Check sheet for the modelled part. Datum: model origin and axes. Units: mm. A direction names the side the tool comes from. Round coordinates to 2 decimals unless told otherwise and drop trailing zeros. Write each loop counter-clockwise with the first axis right and the second up, starting at its lowest first coordinate (ties: lowest second). Pieces come first, ordered by that corner, then holes.
Item 1: Tool access check on faces 5 (the flat face through (-44, 66, -115)), 6 (the flat face through (2, 173, 115)), 7 (the flat face through (-195.247, -51.359, 90.437)), 8 (the flat face through (195.247, -50.911, 90.437)), 9 (the flat face through (2.381, -89.352, 84.531)). Record the directions out of +Z, -Z, +X, -X, +Y, -Y that give a thin tool (end or side, any length) a straight path to the whole face; none if there is none.
Item 2: Go/stop test with flat-tipped pins: pin 1 Ø12 at (y, z) = (275, -32.5) entering from -X; pin 2 Ø6 at (y, z) = (141.5, 30.5) entering from +X; pin 3 Ø11.5 at (x, y) = (-20.5, -47) entering from +Z. Record where each tip stops, or that it passes through.
Item 3: Material ranges on line 1 (Y direction, x = 0, z = -46); line 2 (X direction, y = -46, z = -49); line 3 (Z direction, x = -53.5, y = -56), recorded low to high.
Item 4: Cross-section at D-D on z = 44.5. Enter the section's corners in (x, y), plus the area to 3 significant figures.
Item 5: Cross-section at B-B on z = -22.5. Enter the section's corners in (x, y), plus the area to 3 significant figures.
Item 6: Cross-section at A-A on z = -49. Enter the section's corners in (x, y), plus the area to 3 significant figures.
Item 7: Cross-section at C-C on z = 88. Enter the section's corners in (x, y).
Item 8: Release check for a two-part mould opening along X. For faces 1 (the flat face through (2, -110.03, -25)), 2 (the cylindrical face through (-205.024, -95.772, -25.479)), 3 (the flat face through (225.06, 39, 53)), 4 (the cylindrical face through (10.84, 61.22, -65.7)) record: +X half, -X half, draft (parallel to the pull), parting line (faces both ways), or undercut.
from build123d import *
from OCP.BRepFilletAPI import BRepFilletAPI_MakeChamfer

# Parameters (mm, degrees)
BOSS_EXTRUDE1_DEPTH = 115
CHAMFER3_SIZE       = 60
CHAMFER3_SIZE2      = 42.012452293
FILLET1_R           = 10
SKETCH2_R           = 88.57
BOSS_EXTRUDE2_DEPTH = 225.06
SKETCH3_R           = 50
CUT_EXTRUDE1_DEPTH  = 100


with BuildPart() as part:
    # Sketch1 → Boss-Extrude1 (new, symmetric)
    with BuildSketch(Plane.XY):
        with BuildLine():
            ThreePointArc((-220.06, 110.03), (0, 330.09), (220.06, 110.03))
            Line((220.06, 110.03), (-220.06, 110.03))
        make_face()
        with BuildLine():
            ThreePointArc((-170.06, -110.03), (-205.415339059, -95.385339059), (-220.06, -60.03))
            Line((-220.06, -60.03), (-220.06, 110.03))
            Line((-220.06, 110.03), (220.06, 110.03))
            Line((220.06, 110.03), (220.06, -60.03))
            ThreePointArc((220.06, -60.03), (205.415339059, -95.385339059), (170.06, -110.03))
            Line((170.06, -110.03), (-170.06, -110.03))
        make_face()
    extrude(amount=BOSS_EXTRUDE1_DEPTH, both=True)

    # Chamfer3: one chamfer whose edges measure the first distance from different faces: ONE call of the kernel's chamfer builder (chamfer() names one face for all edges)
    chamfer3_edges_1 = [part.edges().sort_by_distance(p)[0] for p in [
        (-220.06, 25, 115),
    ]]
    chamfer3_side_1 = [part.faces().sort_by_distance(p)[0] for p in [
        (-220.06, 25, 0),
    ]]
    chamfer3_edges_2 = [part.edges().sort_by_distance(p)[0] for p in [
        (-205.415339059, -95.385339059, 115),
    ]]
    chamfer3_side_2 = [part.faces().sort_by_distance(p)[0] for p in [
        (-205.415339059, -95.385339059, 0),
    ]]
    chamfer3_edges_3 = [part.edges().sort_by_distance(p)[0] for p in [
        (0, -110.03, 115),
    ]]
    chamfer3_side_3 = [part.faces().sort_by_distance(p)[0] for p in [
        (0, -110.03, 0),
    ]]
    chamfer3_edges_4 = [part.edges().sort_by_distance(p)[0] for p in [
        (205.415339059, -95.385339059, 115),
    ]]
    chamfer3_side_4 = [part.faces().sort_by_distance(p)[0] for p in [
        (205.415339059, -95.385339059, 0),
    ]]
    chamfer3_edges_5 = [part.edges().sort_by_distance(p)[0] for p in [
        (220.06, 25, 115),
    ]]
    chamfer3_side_5 = [part.faces().sort_by_distance(p)[0] for p in [
        (220.06, 25, 0),
    ]]
    chamfer3_edges_6 = [part.edges().sort_by_distance(p)[0] for p in [
        (0, 330.09, 115),
    ]]
    chamfer3_side_6 = [part.faces().sort_by_distance(p)[0] for p in [
        (0, 330.09, 0),
    ]]
    chamfer3 = BRepFilletAPI_MakeChamfer(part.part.solid().wrapped)
    for e in chamfer3_edges_1:
        chamfer3.Add(CHAMFER3_SIZE, CHAMFER3_SIZE2, e.wrapped, chamfer3_side_1[0].wrapped)  # the first distance lies on this face
    for e in chamfer3_edges_2:
        chamfer3.Add(CHAMFER3_SIZE, CHAMFER3_SIZE2, e.wrapped, chamfer3_side_2[0].wrapped)  # the first distance lies on this face
    for e in chamfer3_edges_3:
        chamfer3.Add(CHAMFER3_SIZE, CHAMFER3_SIZE2, e.wrapped, chamfer3_side_3[0].wrapped)  # the first distance lies on this face
    for e in chamfer3_edges_4:
        chamfer3.Add(CHAMFER3_SIZE, CHAMFER3_SIZE2, e.wrapped, chamfer3_side_4[0].wrapped)  # the first distance lies on this face
    for e in chamfer3_edges_5:
        chamfer3.Add(CHAMFER3_SIZE, CHAMFER3_SIZE2, e.wrapped, chamfer3_side_5[0].wrapped)  # the first distance lies on this face
    for e in chamfer3_edges_6:
        chamfer3.Add(CHAMFER3_SIZE, CHAMFER3_SIZE2, e.wrapped, chamfer3_side_6[0].wrapped)  # the first distance lies on this face
    add(Compound.cast(chamfer3.Shape()), mode=Mode.REPLACE)

    # Fillet1
    fillet1_edges = [part.edges().sort_by_distance(p)[0] for p in [
        (0, 330.09, -115),
        (220.06, 25, 55),
        (0, 288.077547707, 115),
        (-178.047547707, 25, 115),
        (-175.708049149, -65.678049149, 115),
        (0, -68.017547707, 115),
        (175.708049149, -65.678049149, 115),
        (178.047547707, 25, 115),
        (205.415339059, -95.385339059, 55),
        (0, -110.03, 55),
        (-205.415339059, -95.385339059, 55),
        (-220.06, 25, 55),
        (0, 330.09, 55),
        (220.06, 25, -115),
        (205.415339059, -95.385339059, -115),
        (0, -110.03, -115),
        (-205.415339059, -95.385339059, -115),
        (-220.06, 25, -115),
    ]]
    fillet(fillet1_edges, radius=FILLET1_R)

    # Sketch2 → Boss-Extrude2 (add, symmetric)
    with BuildSketch(Plane(origin=(0, 0, 0), x_dir=(0, 0, -1), z_dir=(1, 0, 0))):
        with Locations((-51.847012111, 38.15)):
            Circle(SKETCH2_R)
    extrude(amount=BOSS_EXTRUDE2_DEPTH, both=True)

    # Sketch3 → Cut-Extrude1 (cut)
    with BuildSketch(Plane(origin=(0, 0, -115), x_dir=(-1, 0, 0), z_dir=(0, 0, -1))):
        with Locations((0, 110.03)):
            Circle(SKETCH3_R)
    extrude(amount=-CUT_EXTRUDE1_DEPTH, mode=Mode.SUBTRACT)


solid = part.part
Response values:
1. face 5: -Z, +X, -X, +Y, -Y
1. face 6: +Z, +X, -X, +Y
1. face 7: +Z, -X, -Y
1. face 8: +Z, +X, -Y
1. face 9: +Z, +X, -X, -Y
2. pin 1: stops at x = -152.17
2. pin 2: stops at x = 218.21
2. pin 3: stops at z = 115
3. line 1: y = -110.03 to 60.03, 160.03 to 330.09
3. line 2: x = -220.06 to 220.06
3. line 3: z = -115 to 115
4. outline: (-225.06, -50.11) - (-220.06, -50.11) - (-220.06, -60.03) arc R50 ccw to (-170.06, -110.03) - (170.06, -110.03) arc R50 ccw to (220.06, -60.03) - (220.06, -50.11) - (225.06, -50.11) - (225.06, 126.41) - (219.45, 126.41) arc R220.06 ccw to (-219.45, 126.41) - (-225.06, 126.41) - close
4. area: 174,000 mm2
5. outline: (-225.06, -9.99) - (-220.06, -9.99) - (-220.06, -60.03) arc R50 ccw to (-170.06, -110.03) - (170.06, -110.03) arc R50 ccw to (220.06, -60.03) - (220.06, -9.99) - (225.06, -9.99) - (225.06, 86.29) - (220.06, 86.29) - (220.06, 110.03) arc R220.06 ccw to (-220.06, 110.03) - (-220.06, 86.29) - (-225.06, 86.29) - close; hole circle Ø100 at (0, 110.03)
5. area: 165,000 mm2
6. outline: (-220.06, -60.03) arc R50 ccw to (-170.06, -110.03) - (170.06, -110.03) arc R50 ccw to (220.06, -60.03) - (220.06, 110.03) arc R220.06 ccw to (-220.06, 110.03) - close; hole circle Ø100 at (0, 110.03)
6. area: 164,000 mm2
7. outline: (-225.06, -42.71) - (-196.95, -42.71) - (-196.95, -60.03) arc R26.89 ccw to (-170.06, -86.92) - (170.06, -86.92) arc R26.89 ccw to (196.95, -60.03) - (196.95, -42.71) - (225.06, -42.71) - (225.06, 119.01) - (196.75, 119.01) arc R196.95 ccw to (-196.75, 119.01) - (-225.06, 119.01) - close
8. face 1: draft
8. face 2: -X half
8. face 3: +X half
8. face 4: undercut
